Here's how the part is built. I have some questions about the finished solid (model axes, mm). A direction names the side the tool comes from. Round coordinates to 2 decimals unless told otherwise and drop trailing zeros. Order: outer loops, then holes, each group sorted by start corner. A loop starts at its lowest first (then second) coordinate and runs counter-clockwise, first axis right, second up. Notation, with made-up numbers: (-37.75, 37) -> (21.25, 37) arc R21 ccw to (21.25, 50) -> close; hole circle Ø2 at (28.25, -35). An arc over 180 degrees is marked (long way). Use a Markdown table: item, result. Add a question column.
(1) I want a section at D-D, the plane x = 47. Please give me the cut outline in (y, z).
(2) I want a section at C-C, the plane y = 5.5. Give the number of separate pieces and of enclosed holes in the cut face, then the cut area to 3 significant figures.
(3) On a 3-axis mill with a long thin cutter (end or side, diameter ignored), from which of +Z, -Z, +X, -X, +Y, -Y can I reach the whole of each face in a straight line? I mean faces 4 (the face through (2.2, 7.8, -83.8)), 5 (the face through (-2.828, 1.232, -2.603)), 6 (the face through (-4.005, 6, -46)). Say none if no direction works.
(4) I'm going to push flat-ended pins straight in: P1, Ø3, axis at x = 80.45, z = -3.99, coming from the +Y side; P2, Ø1.7, axis at x = 81.5, z = -3.5, coming from the -Y side; P3, Ø2, axis at x = 28.5, z = -17.5, coming from the +Y side. Where does each tip first touch, or does it pass through?
(5) Thinking about a two-plate mould opening in X: for faces 1 (the face through (83, 12.8, -28)), 2 (the face through (83.14, 6.49, -89.04)), 3 (the face through (1, 2.5, -88)), which applies, pulls with the +X half, pulls with the -X half, needs draft (parallel to the pull), parting line crosses it, or undercut?
(6) If I drill on probe 1 along X at (y, z) = (11.25, -73); probe 2 along Z at (x, y) = (60, 4); probe 3 along Z at (x, y) = (79.5, 6.75), over which ranges is the centre line in solid material (lowest first)?
(7) I want a section at B-B, the plane z = -37.5. Please give me the cut outline in (x, y).
(8) I want a section at A-A, the plane x = 67. Please give me the cut outline in (y, z), then the cut area to 3 significant figures.
Autodesk Inventor part; units mm, degrees
ref_plane "YZ Plane" through (0, 0, 0) normal (1, 0, 0) x (0, 1, 0)
ref_plane "XZ Plane" through (0, 0, 0) normal (0, 1, 0) x (-1, 0, 0)
ref_plane "XY Plane" through (0, 0, 0) normal (0, 0, 1) x (1, 0, 0)
sketch "bottom" plane through (0, 0, 0) normal (0, 1, 0) x (-1, 0, 0)
  line L0 (4.0046, -0.4434) -> (-83.9954, -0.4434)
  line L1 (-83.9954, -0.4434) -> (-83.9954, -89.9434)
  line L2 (-83.9954, -89.9434) -> (4.0046, -89.9434)
  line L3 (4.0046, -89.9434) -> (4.0046, -0.4434)
  line L4 (2.2046, -2.2434) -> (-82.1954, -2.2434)
  line L5 (-82.1954, -2.2434) -> (-82.1954, -88.1434)
  line L6 (-82.1954, -88.1434) -> (2.2046, -88.1434)
  line L7 (2.2046, -88.1434) -> (2.2046, -2.2434)
  circle A0 centre (0.4546, -3.9934) radius 3.55
  line L8 (-39.9954, -123.8489) -> (-39.9954, 33.4211)
  line L9 (23.3841, -45.1934) -> (-117.3219, -45.1934)
  circle A1 centre (0.4546, -3.9934) radius 1.75
  circle A2 centre (-80.4454, -3.9934) radius 3.55
  circle A3 centre (-80.4454, -3.9934) radius 1.75
  circle A4 centre (0.4546, -86.3934) radius 1.75
  circle A5 centre (0.4546, -86.3934) radius 3.55
  circle A6 centre (-80.4454, -86.3934) radius 1.75
  circle A7 centre (-80.4454, -86.3934) radius 3.55
  line L10 (3.6301, -3.9991) -> (2.0374, -6.7462)
  line L11 (2.0374, -6.7462) -> (-1.138, -6.7405)
  line L12 (-1.138, -6.7405) -> (-2.7208, -3.9877)
  line L13 (-2.7208, -3.9877) -> (-1.1282, -1.2406)
  line L14 (-1.1282, -1.2406) -> (2.0472, -1.2462)
  line L15 (2.0472, -1.2462) -> (3.6301, -3.9991)
  circle A8 centre (0.4546, -3.9934) radius 4.55
  point P0 (0, 0)
  point P1 (-39.9954, -45.1934)
  point P2 (-2.6341, -2.2434)
  point P3 (2.2046, -7.0821)
  point P4 (2.2046, -83.3047)
  point P5 (-2.6341, -88.1434)
  point P6 (-77.3567, -88.1434)
  point P7 (-82.1954, -83.3047)
  point P8 (-82.1954, -7.0821)
  point P9 (-77.3567, -2.2434)
  point P10 (-39.9954, -0.4434)
  point P11 (-39.9954, -2.2434)
  point P12 (2.2046, -45.1934)
  point P13 (4.0046, -45.1934)
  point P14 (-39.9954, -45.1934)
  point P15 (-3.7454, -2.2434)
  point P16 (2.2046, -8.1934)
  dimension "d0" = 88
  dimension "d1" = 89.5
  dimension "d2" = 84.4
  dimension "d3" = 85.9
  dimension "d4" = 1.8
  dimension "d5" = 1.8
  dimension "d6" = 7.1
  dimension "d7" = 3.55
  dimension "d8" = 3.55
  dimension "d9" = 3.5
  dimension "d10" = 88
  dimension "d11" = 89.5
  dimension "d12" = 44.75
  dimension "d13" = 44
  dimension "d33" = 2.75
  dimension "d36" = 9.1
ref_plane "Work Plane3" through (39.9954, 0, -45.1934) normal (0, 0, 1) x (1, 0, 0)
ref_plane "Work Plane4" through (39.9954, 0, -45.1934) normal (1, 0, 0) x (0, 1, 0)
extrude "Extrusion4" add sketch "bottom" along normal blind 12.8 contours L3 A8 L0 | A8 L3 A0 L0 | A0 L4 A8 L0 | A0 L7 L10 L15 L14 L13 L4 | A8 L4 L8 L0 | L3 A8 L7 A0 | L4 L13 L12 L11 L10 L7 A0 | L3 L9 L7 A8 | L13 L14 L15 L10 L7 L4 | L4 A1 L7 L10 L11 L12 L13 | L4 L7 A1
extrude "Extrusion5" add sketch "bottom" along normal blind 1.8 contours A0 L7 A8 L4 | A8 L7 L9 L8 L4
fillet "Fillet3" radius 3 1 edges at (-4.0046, 6.4, -0.4434)
fillet "Fillet4" radius 1.5 2 edges at (-2.2046, 7.3, -7.0821) (2.6341, 7.3, -2.2434)
extrude "Extrusion6" cut sketch "bottom" along normal blind 2.5 contours L13 L14 L15 L10 L7 L4 | L4 A1 L7 L10 L11 L12 L13 | L4 L7 A1
extrude "pcb hight" add sketch "bottom" along normal blind 7.8 contours A0 L7 A8 L4
mirror "Mirror3" about plane through (39.9954, 0, -45.1934) normal (0, 0, 1)
mirror "Mirror4" about plane through (39.9954, 0, -45.1934) normal (1, 0, 0)
sketch "Sketch4" plane through (-1.0046, 0, -0.4434) normal (0, 0, 1) x (1, 0, 0)
  line L0 (65.6777, 7.8088) -> (75.6777, 7.8088)
  line L1 (75.6777, 7.8088) -> (75.6777, 4.3088)
  line L2 (75.6777, 4.3088) -> (65.6777, 4.3088)
  line L3 (65.6777, 4.3088) -> (65.6777, 7.8088)
  point P0 (1.0046, 0)
  dimension "d39" = 10
  dimension "d40" = 3.5
extrude "Extrusion8" cut sketch "Sketch4" against normal blind 1.8
equation "\"d2\" = d0 - 2 * d4"
equation "\"d3\" = d1 - 2 * d5"
equation "\"d5\" = d4"
equation "\"d6\" = 2 * d4 + d9"
equation "\"d7\" = 0.5 * d6"
equation "\"d8\" = 0.5 * d6"
equation "\"d10\" = d0"
equation "\"d11\" = d1"
equation "\"d29\" = d4"
properties part number "base"
Taken from the geometry:
| question | item | result |
|---|---|---|
| 1 | outline | (0, -89.94) -> (12.8, -89.94) -> (12.8, -88.14) -> (1.8, -88.14) -> (1.8, -2.24) -> (12.8, -2.24) -> (12.8, -0.44) -> (0, -0.44) -> close |
| 2 | separate pieces | 1 |
| 2 | enclosed holes | 4 |
| 2 | area | 702 mm2 |
| 3 | face 4 | +Y |
| 3 | face 5 | -Y |
| 3 | face 6 | +Z, -Z, -X, +Y, -Y |
| 4 | P1 | passes through |
| 4 | P2 | stops at y = 2.5 |
| 4 | P3 | stops at y = 1.8 |
| 5 | face 1 | needs draft |
| 5 | face 2 | pulls with the +X half |
| 5 | face 3 | undercut |
| 6 | probe 1 | x = -4 to -2.2, 82.2 to 84 |
| 6 | probe 2 | z = -89.94 to -88.14, -2.24 to -0.44 |
| 6 | probe 3 | z = -89.94 to -87.87, -84.92 to -81.94, -8.44 to -5.47, -2.52 to -0.44 |
| 7 | outline | (-4, 0) -> (84, 0) -> (84, 12.8) -> (82.2, 12.8) -> (82.2, 1.8) -> (-2.2, 1.8) -> (-2.2, 12.8) -> (-4, 12.8) -> close |
| 8 | outline | (0, -89.94) -> (12.8, -89.94) -> (12.8, -88.14) -> (1.8, -88.14) -> (1.8, -2.24) -> (4.31, -2.24) -> (4.31, -0.44) -> (0, -0.44) -> close; (7.81, -2.24) -> (12.8, -2.24) -> (12.8, -0.44) -> (7.81, -0.44) -> close |
| 8 | area | 194 mm2 |
